Input: dimensioned drawing with shaded views. Units: mm. Origin: part minimum x, y, z. Give positions to 0.01 mm unless a question says otherwise; leave off trailing zeros. Loops run counter-clockwise (first coordinate to the right, second up) from the corner with the lowest first, then second, coordinate; pieces in that order, holes last.
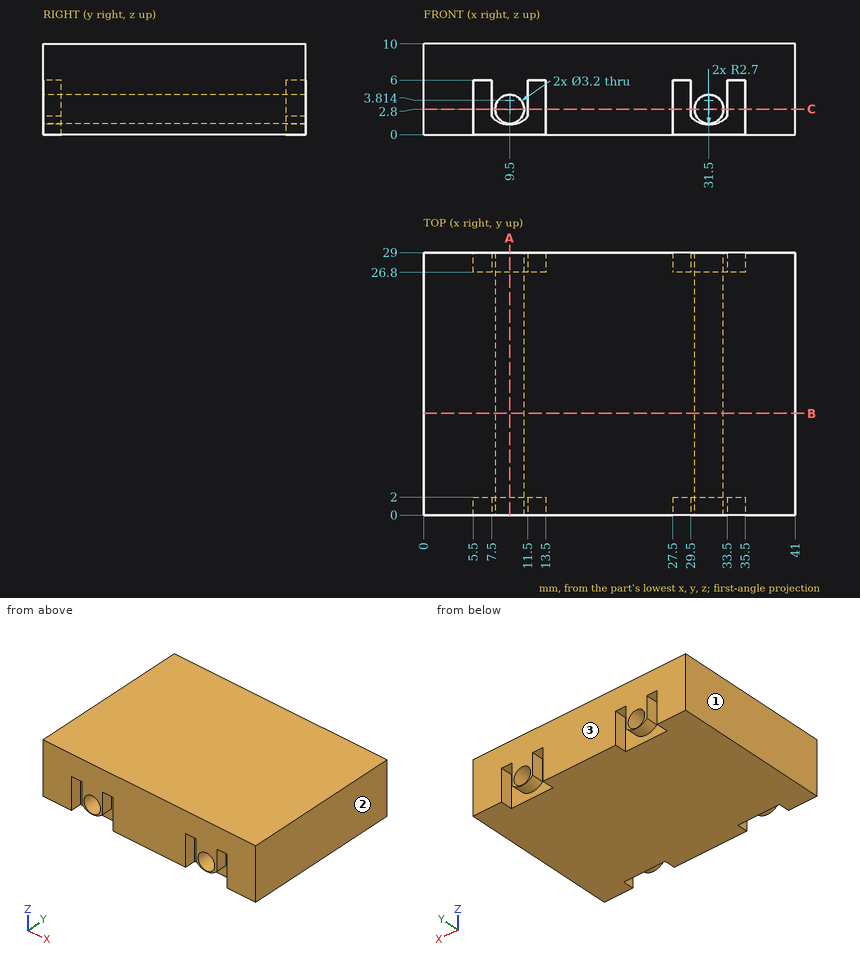
(1) Section A-A, the plane x = 9.5. Return the cut outline in (y, z).
A:
outline: (0, 1.11) - (2, 1.11) - (2, 0) - (26.8, 0) - (26.8, 1.11) - (29, 1.11) - (29, 1.2) - (0, 1.2) - close; (0, 4.4) - (29, 4.4) - (29, 10) - (0, 10) - close
(2) Section B-B, the plane y = 11.25. Return the cut outline in (x, z), then the cut area to 3 significant figures.
A:
outline: (0, 0) - (41, 0) - (41, 10) - (0, 10) - close; hole circle Ø3.2 at (9.5, 2.8); hole circle Ø3.2 at (31.5, 2.8)
area: 394 mm2
(3) Ray query, line 1 along X through (y, z) = (10.25, 2.8); line 2 along Z through (x, y) = (9.5, 12.5); line 3 along Y through (x, z) = (7.5, 1.5). Return the intervals inside material, ascending.
A:
line 1: x = 0 to 7.9, 11.1 to 29.9, 33.1 to 41
line 2: z = 0 to 1.2, 4.4 to 10
line 3: y = 2 to 26.8
(4) Section C-C, the plane z = 2.8. Count the separate pieces of the cut face and the enclosed holes in it, then the cut area to 3 significant figures.
A:
separate pieces: 3
enclosed holes: 0
area: 970 mm2
(5) Mould query, pull axis X, two halves, no side actions, for the marked faces 1, 2 and 3. Classes: pulls with the +X half, pulls with the -X half, needs draft (parallel to the pull), parting line crosses it, or undercut.
A:
face 1: pulls with the -X half
face 2: pulls with the +X half
face 3: needs draft
(6) First-contact query: pin 1 (0.6 mm diameter, centred on x = 12.5, y = 27.5, fed in from -Z); pin 2 (2.5 mm diameter, centred on x = 9.5, z = 2.8, fed in from -Y). Flat tips, straight axial feed; report the tip coordinate or a pass-through.
A:
pin 1: stops at z = 6
pin 2: passes through
